For this review, take the finished solid that the model builds, in its own axes (mm). Face numbers are marked on the shaded views. Coordinates: 2 decimals unless noted, no trailing zeros. Loops run counter-clockwise (first coordinate to the right, second up) from the corner with the lowest first, then second, coordinate; pieces in that order, holes last. Notation, with made-up numbers: M -23.75,29.25 L 4.25,29.25 A19 cw 4.25,34.25 Z; hole C 9.25,-23 d3. An arc over 180 degrees is marked long. Answer as a JSON object with one key per item and string values. Group by question number.
Item 1: Wall thickness on L1, parallel to X at y = 1.5, z = 17; L2, parallel to Y at x = -7.5, z = 10.75; L3, parallel to Y at x = -2, z = 17.5: over which ranges is each line inside the solid? List them lowest first. Write a range as from..to.
Item 2: Insertion check: pin 1 (6 mm diameter, centred on x = -3.32, y = 1.93, fed in from +Z). The pin has a flat end and moves straight along its axis. Give the tip position at first contact, or say it passes through.
Item 3: Add section A-A (z = 8). State the section outline as (x, y) points, then the cut area to 3 significant figures.
Item 4: Mouldability with a two-part tool opening along X and no side actions: class the marked faces 1, 2 and 3 as +X half, -X half, draft (parallel to the pull), parting line (faces both ways), or undercut.
Item 5: Add section B-B (z = 16). State the section outline as (x, y) points.
from build123d import *

# Parameters (mm, degrees)
F0_W     = 20
F0_H     = 20
F1_DEPTH = 20
F3_D     = 10
F3_DEPTH = 10
F3_TIP   = 3.0043030951


with BuildPart() as f1:
    # F0 (on Top) → F1 (new body)
    with BuildSketch(Plane.XY):
        with Locations((-3.3169160597, 1.9259513356)):
            Rectangle(F0_W, F0_H)
    extrude(amount=F1_DEPTH)

    # F3
    with Locations(Plane.XY.offset(20)):
        with Locations((-3.3169160597, 1.9259513356)):
            Hole(F3_D / 2, depth=F3_DEPTH)
            with Locations((0, 0, -(F3_DEPTH + F3_TIP / 2))):  # 118° drill point
                Cone(0, F3_D / 2, F3_TIP, mode=Mode.SUBTRACT)


solid = f1.part
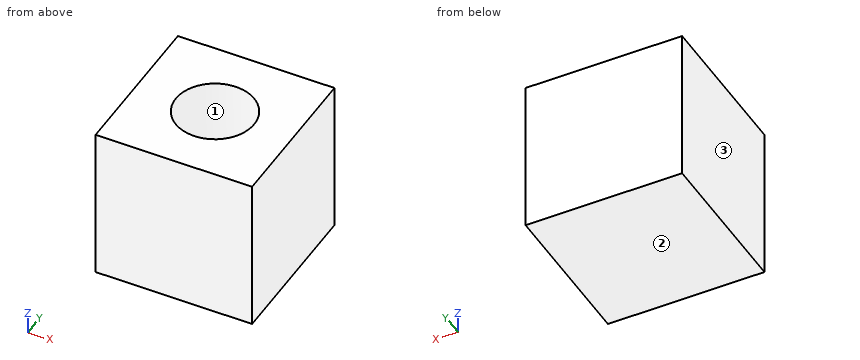
From the geometry:
{
 "1": {"L1": "x = -13.32..-8.3, 1.66..6.68", "L2": "y = -8.07..-0.81, 4.66..11.93", "L3": "y = -8.07..-2.9, 6.75..11.93"},
 "2": {"pin 1": "stops at z = 8.8"},
 "3": {"outline": "M -13.32,-8.07 L 6.68,-8.07 L 6.68,11.93 L -13.32,11.93 Z; hole C -3.32,1.93 d3.34", "area": "391 mm²"},
 "4": {"face 1": "undercut", "face 2": "draft", "face 3": "-X half"},
 "5": {"outline": "M -13.32,-8.07 L 6.68,-8.07 L 6.68,11.93 L -13.32,11.93 Z; hole C -3.32,1.93 d10"}
}
